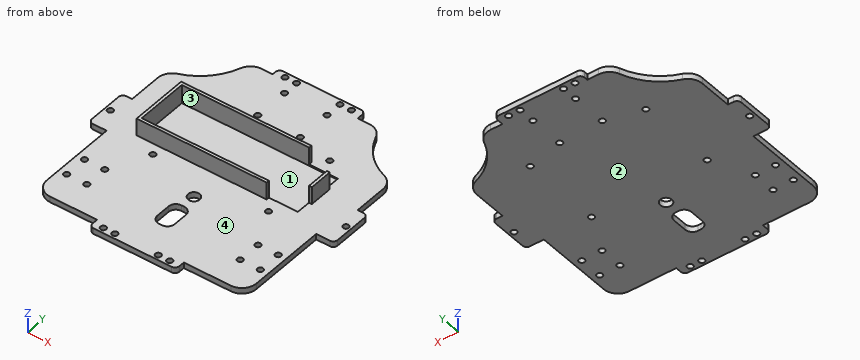
from build123d import *

# Parameters (mm, degrees)
BOSS_EXTRUDE1_DEPTH = 4
SKETCH2_R           = 2
SKETCH2_R_2         = 4
CUT_EXTRUDE1_DEPTH  = 5
BOSS_EXTRUDE2_DEPTH = 12
SKETCH5_W           = 108
SKETCH5_H           = 36
CUT_EXTRUDE3_DEPTH  = 13


with BuildPart() as part:
    # Sketch1 → Boss-Extrude1 (new body)
    with BuildSketch(Plane.XY):
        with BuildLine():
            Line((82, 15), (78, 15))
            Line((78, 15), (78, 37.978728218))
            ThreePointArc((78, 37.978728218), (76.185352772, 43.723290865), (71.4, 47.382982574))
            ThreePointArc((71.4, 47.382982574), (56.923524203, 56.509448815), (47.586109287, 70.850767451))
            ThreePointArc((47.586109287, 70.850767451), (43.91712949, 75.540642349), (38.232636609, 77.313459314))
            Line((38.232636609, 77.313459314), (30, 77.313459314))
            Line((30, 77.313459314), (30, 81.313459314))
            ThreePointArc((30, 81.313459314), (29.121320344, 83.434779658), (27, 84.313459314))
            Line((27, 84.313459314), (-27, 84.313459314))
            ThreePointArc((-27, 84.313459314), (-29.121320344, 83.434779658), (-30, 81.313459314))
            Line((-30, 81.313459314), (-30, 78.861186474))
            Line((-30, 78.861186474), (-37.676235378, 78.861186474))
            ThreePointArc((-37.676235378, 78.861186474), (-43.495271937, 76.993763774), (-47.140988303, 72.08894918))
            ThreePointArc((-47.140988303, 72.08894918), (-56.458737454, 56.975076587), (-71.4, 47.382982574))
            ThreePointArc((-71.4, 47.382982574), (-76.185352772, 43.723290865), (-78, 37.978728218))
            Line((-78, 37.978728218), (-78, 15))
            Line((-78, 15), (-82, 15))
            ThreePointArc((-82, 15), (-84.121320344, 14.121320344), (-85, 12))
            Line((-85, 12), (-85, -12))
            ThreePointArc((-85, -12), (-84.121320344, -14.121320344), (-82, -15))
            Line((-82, -15), (-72.5, -15))
            Line((-72.5, -15), (-72.5, -68.686540686))
            ThreePointArc((-72.5, -68.686540686), (-69.571067812, -75.757608498), (-62.5, -78.686540686))
            Line((-62.5, -78.686540686), (-30, -78.686540686))
            Line((-30, -78.686540686), (-30, -82.686540686))
            ThreePointArc((-30, -82.686540686), (-29.121320344, -84.807861029), (-27, -85.686540686))
            Line((-27, -85.686540686), (27, -85.686540686))
            ThreePointArc((27, -85.686540686), (29.121320344, -84.807861029), (30, -82.686540686))
            Line((30, -82.686540686), (30, -78.686540686))
            Line((30, -78.686540686), (62.5, -78.686540686))
            ThreePointArc((62.5, -78.686540686), (69.571067812, -75.757608498), (72.5, -68.686540686))
            Line((72.5, -68.686540686), (72.5, -15))
            Line((72.5, -15), (82, -15))
            ThreePointArc((82, -15), (84.121320344, -14.121320344), (85, -12))
            Line((85, -12), (85, 12))
            ThreePointArc((85, 12), (84.121320344, 14.121320344), (82, 15))
        make_face()
    extrude(amount=BOSS_EXTRUDE1_DEPTH)

    # Sketch2 → Cut-Extrude1 (cut)
    with BuildSketch(Plane.XY.offset(4)):
        with Locations((81.5, 0)):
            Circle(SKETCH2_R)
        with Locations((-81.5, 0)):
            Circle(SKETCH2_R)
        with Locations((15, 80.813459314)):
            Circle(SKETCH2_R)
        with Locations((23, 80.813459314)):
            Circle(SKETCH2_R)
        with Locations((-23, 80.813459314)):
            Circle(SKETCH2_R)
        with Locations((-15, 80.813459314)):
            Circle(SKETCH2_R)
        with Locations((-23, -82.186540686)):
            Circle(SKETCH2_R)
        with Locations((-15, -82.186540686)):
            Circle(SKETCH2_R)
        with Locations((15, -82.186540686)):
            Circle(SKETCH2_R)
        with Locations((23, -82.186540686)):
            Circle(SKETCH2_R)
        with Locations((67, -42)):
            Circle(SKETCH2_R)
        with Locations((67, -58)):
            Circle(SKETCH2_R)
        with Locations((-40, -15.686540686)):
            Circle(SKETCH2_R)
        with Locations((40, -15.686540686)):
            Circle(SKETCH2_R)
        with Locations((40, 39.313459314)):
            Circle(SKETCH2_R)
        with Locations((-40, 39.313459314)):
            Circle(SKETCH2_R)
        with Locations((0, -30.686540686)):
            Circle(SKETCH2_R_2)
        with Locations((-15, 70.007888798)):
            Circle(SKETCH2_R)
        with Locations((15, 69.313459314)):
            Circle(SKETCH2_R)
        with Locations((-15, 46.007888798)):
            Circle(SKETCH2_R)
        with Locations((15, 45.313459314)):
            Circle(SKETCH2_R)
        with Locations((53, -58)):
            Circle(SKETCH2_R)
        with Locations((53, -42)):
            Circle(SKETCH2_R)
        with Locations((-53, -58)):
            Circle(SKETCH2_R)
        with Locations((-67, -58)):
            Circle(SKETCH2_R)
        with Locations((-67, -42)):
            Circle(SKETCH2_R)
        with Locations((-53, -42)):
            Circle(SKETCH2_R)
        with BuildLine():
            Line((-1, -40.686540686), (1, -40.686540686))
            ThreePointArc((1, -40.686540686), (4.535533906, -42.15100678), (6, -45.686540686))
            Line((6, -45.686540686), (6, -55.686540686))
            ThreePointArc((6, -55.686540686), (4.535533906, -59.222074592), (1, -60.686540686))
            Line((1, -60.686540686), (-1, -60.686540686))
            ThreePointArc((-1, -60.686540686), (-4.535533906, -59.222074592), (-6, -55.686540686))
            Line((-6, -55.686540686), (-6, -45.686540686))
            ThreePointArc((-6, -45.686540686), (-4.535533906, -42.15100678), (-1, -40.686540686))
        make_face()
    extrude(amount=-CUT_EXTRUDE1_DEPTH, mode=Mode.SUBTRACT)

    # Sketch3 → Boss-Extrude2 (add)
    with BuildSketch(Plane.XY.offset(4)):
        Polygon((-57, -8.186540686), (33, -8.186540686), (33, -6.186540686), (53, -6.186540686), (53, 3.813459314), (55, 3.813459314), (55, 19.813459314), (53, 19.813459314), (53, 29.813459314), (33, 29.813459314), (33, 31.813459314), (-57, 31.813459314), align=None)
    extrude(amount=BOSS_EXTRUDE2_DEPTH)

    # Sketch5 → Cut-Extrude3 (cut)
    with BuildSketch(Plane.XY.offset(16)):
        with Locations((-1, 11.813459314)):
            Rectangle(SKETCH5_W, SKETCH5_H)
    extrude(amount=-CUT_EXTRUDE3_DEPTH, mode=Mode.SUBTRACT)


solid = part.part
CAD build for the part. Positions are in the model's coordinates, mm. Face numbers are marked on the shaded views. A direction names the side the tool comes from. Round coordinates to 2 decimals unless told otherwise and drop trailing zeros. Write each loop counter-clockwise with the first axis right and the second up, starting at its lowest first coordinate (ties: lowest second). Pieces come first, ordered by that corner, then holes.
(1) Mould opens along Y. For the marked faces 3 and 4 say: pulls with the +Y half, pulls with the -Y half, needs draft (parallel to the pull), parting line crosses it, or undercut.
(2) 3-axis set-ups, long thin cutter, end or side, ignore diameter. For the marked faces 1 and 2: which of +Z, -Z, +X, -X, +Y, -Y reach the whole face in a straight line?
(3) Slice it at B-B, the plane z = 7.75. Write the cut outline in (x, y).
(4) Probe line 1 along Y through (x, z) = (15, 2.6); line 2 along Y through (x, z) = (-23, 1); line 3 along Y through (x, z) = (11.5, 9.25). List the from-to ranges inside material, lowest first.
(5) Slice it at D-D, the plane y = -58. Write the cut outline in (x, z).
(6) Slice it at A-A, the plane x = 23. Write the cut outline in (y, z).
(7) Drop flat-ended pins along their axis: P1, Ø4, axis at x = -46, y = -28, coming from the +Z side; P2, Ø0.6, axis at x = 54, z = 8, coming from the -Y side; P3, Ø1.2, axis at x = -76.5, z = 3, coming from the -Y side. Give the stop position or say it passes through.
(8) Slice it at C-C, the plane x = -15. Write the cut outline in (y, z).
From the geometry:
1. face 3: undercut
1. face 4: needs draft
2. face 1: +Z
2. face 2: -Z, +X, -X, +Y, -Y
3. outline: (-57, -8.19) - (33, -8.19) - (33, -6.19) - (-55, -6.19) - (-55, 29.81) - (33, 29.81) - (33, 31.81) - (-57, 31.81) - close; (53, 3.81) - (55, 3.81) - (55, 19.81) - (53, 19.81) - close
4. line 1: y = -85.69 to -84.19, -80.19 to 43.31, 47.31 to 67.31, 71.31 to 78.81, 82.81 to 84.31
4. line 2: y = -85.69 to -84.19, -80.19 to 78.81, 82.81 to 84.31
4. line 3: y = -8.19 to -6.19, 29.81 to 31.81
5. outline: (-72.5, 0) - (-69, 0) - (-69, 4) - (-72.5, 4) - close; (-65, 0) - (-55, 0) - (-55, 4) - (-65, 4) - close; (-51, 0) - (-5.43, 0) - (-5.43, 4) - (-51, 4) - close; (5.43, 0) - (51, 0) - (51, 4) - (5.43, 4) - close; (55, 0) - (65, 0) - (65, 4) - (55, 4) - close; (69, 0) - (72.5, 0) - (72.5, 4) - (69, 4) - close
6. outline: (-85.69, 0) - (-84.19, 0) - (-84.19, 4) - (-85.69, 4) - close; (-80.19, 0) - (78.81, 0) - (78.81, 4) - (31.81, 4) - (31.81, 16) - (29.81, 16) - (29.81, 3) - (-6.19, 3) - (-6.19, 16) - (-8.19, 16) - (-8.19, 4) - (-80.19, 4) - close; (82.81, 0) - (84.31, 0) - (84.31, 4) - (82.81, 4) - close
7. P1: stops at z = 4
7. P2: stops at y = 3.81
7. P3: stops at y = -15
8. outline: (-85.69, 0) - (-84.19, 0) - (-84.19, 4) - (-85.69, 4) - close; (-80.19, 0) - (44.01, 0) - (44.01, 4) - (31.81, 4) - (31.81, 16) - (29.81, 16) - (29.81, 3) - (-6.19, 3) - (-6.19, 16) - (-8.19, 16) - (-8.19, 4) - (-80.19, 4) - close; (48.01, 0) - (68.01, 0) - (68.01, 4) - (48.01, 4) - close; (72.01, 0) - (78.81, 0) - (78.81, 4) - (72.01, 4) - close; (82.81, 0) - (84.31, 0) - (84.31, 4) - (82.81, 4) - close
